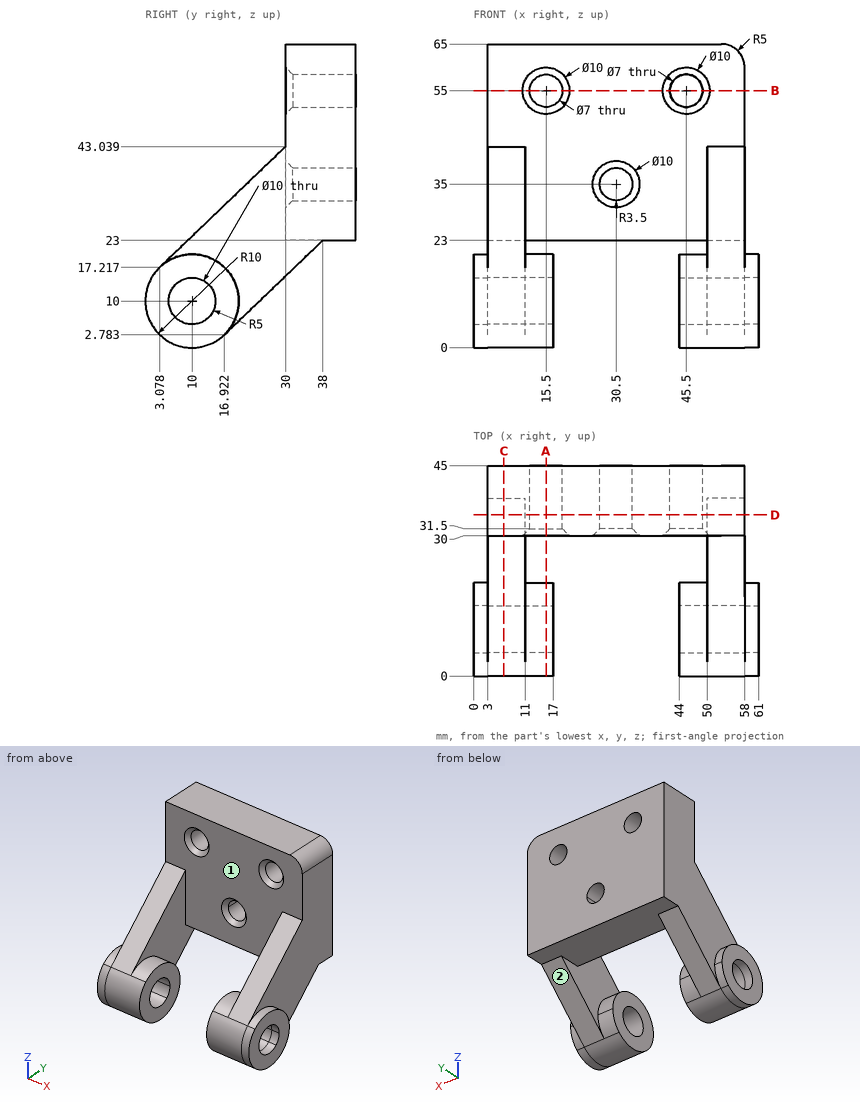
Can you work these out from the drawing? Everything is in mm from the part's minimum corner. A direction names the side the tool comes from. Give positions to 0.01 mm unless a question says otherwise; leave off trailing zeros. Order: outer loops, then holes, each group sorted by start corner. A loop starts at its lowest first (then second) coordinate and runs counter-clockwise, first axis right, second up.
Item 1: I need wall thicknesses on line 1 (Z direction, x = 45.5, y = 38.25); line 2 (Z direction, x = 0.6, y = 10); line 3 (X direction, y = 17, z = 28.5). Which ranges of each line are inside material? Lowest first, please.
Item 2: If we section it at B-B, the plane z = 55: Write out the boundary of the cut face in (x, y).
Item 3: If we section it at D-D, the plane y = 34.5: Write out the boundary of the cut face in (x, z).
Item 4: For the marked faces 1 and 2, which set-ups out of +Z, -Z, +X, -X, +Y, -Y let a thin tool reach every point of the face, with its end or its side?
Item 5: If we section it at A-A, the plane x = 15.5: Write out the boundary of the cut face in (y, z).
Item 6: I'm going to push flat-ended pins straight in: pin 1 (6 mm diameter, centred on x = 53.5, y = 26.5, fed in from +Z); pin 2 (6 mm diameter, centred on x = 26.5, z = 28, fed in from -Y); pin 3 (21 mm diameter, centred on y = 33.5, z = 27, fed in from +X). Where does each tip first touch, or does it pass through?
Item 7: If we section it at C-C, the plane x = 6.5: Write out the boundary of the cut face in (y, z).
Values:
1. line 1: z = 23 to 51.5, 58.5 to 65
1. line 2: z = 0 to 5, 15 to 20
1. line 3: x = 3 to 11, 50 to 58
2. outline: (3, 30) - (10.5, 30) - (12, 31.5) - (12, 45) - (3, 45) - close; (19, 31.5) - (20.5, 30) - (40.5, 30) - (42, 31.5) - (42, 45) - (19, 45) - close; (49, 31.5) - (50.5, 30) - (58, 30) - (58, 45) - (49, 45) - close
3. outline: (3, 19.64) - (11, 19.64) - (11, 23) - (50, 23) - (50, 19.64) - (58, 19.64) - (58, 60) arc R5 ccw to (53, 65) - (3, 65) - close; hole circle Ø7 at (15.5, 55); hole circle Ø7 at (30.5, 35); hole circle Ø7 at (45.5, 55)
4. face 1: +Z, -Y
4. face 2: -Z, +X, -X, +Y
5. outline: circle Ø20 at (10, 10); (30, 23) - (45, 23) - (45, 51.5) - (31.5, 51.5) - (30, 50) - close; (30, 60) - (31.5, 58.5) - (45, 58.5) - (45, 65) - (30, 65) - close; hole circle Ø10 at (10, 10)
6. pin 1: stops at z = 42.56
6. pin 2: stops at y = 30
6. pin 3: stops at x = 58
7. outline: (3.08, 17.22) arc R10 ccw to (16.92, 2.78) - (38, 23) - (45, 23) - (45, 65) - (30, 65) - (30, 43.04) - close; hole circle Ø10 at (10, 10)
